Check sheet for the modelled part. Datum: model origin and axes. Units: mm. A direction names the side the tool comes from. Coordinates: 2 decimals unless noted, no trailing zeros. Loops run counter-clockwise (first coordinate to the right, second up) from the corner with the lowest first, then second, coordinate; pieces in that order, holes last. Notation, with made-up numbers: M 75,17 L 113,17 A22 ccw 113,33 Z; hole C 36.5,-29 d9. An arc over 180 degrees is marked long. Return JSON: item names as keys, results as strings.
from build123d import *

# Parameters (mm, degrees)
SKETCH1_W           = 10.6496793
SKETCH1_H           = 5.5
SKETCH1_W_2         = 3
SKETCH1_H_2         = 45
BOSS_EXTRUDE1_DEPTH = 80
SKETCH2_R           = 2
SKETCH2_R_2         = 1.25
CUT_EXTRUDE1_DEPTH  = 87.830296046
SKETCH3_R           = 5
SKETCH3_R_2         = 1.0922
CUT_EXTRUDE2_DEPTH  = 10
SKETCH4_W           = 28
SKETCH4_H           = 3
SKETCH4_W_2         = 8.5
BOSS_EXTRUDE2_DEPTH = 10.6496793


with BuildPart() as part:
    # Sketch1 → Boss-Extrude1 (new body)
    with BuildSketch(Plane(origin=(0, 0, 0), x_dir=(1, 0, 0), z_dir=(0, 1, 0))):
        with Locations((8.035561223, -6.751971663)):
            Rectangle(SKETCH1_W, SKETCH1_H)
        with Locations((1.210721573, 4.498028337)):
            Rectangle(SKETCH1_W_2, SKETCH1_H_2)
        with Locations((8.035561223, -15.251971663)):
            Rectangle(SKETCH1_W, SKETCH1_H)
    extrude(amount=BOSS_EXTRUDE1_DEPTH)

    # Sketch2 → Cut-Extrude1 (cut, through all)
    with BuildSketch(Plane(origin=(0, 0, 4.001971663), x_dir=(-1, 0, 0), z_dir=(0, 0, -1))):
        with Locations((-7.660400873, 40)):
            Circle(SKETCH2_R)
        with Locations((-7.660400873, 65.273758001)):
            Circle(SKETCH2_R_2)
        with Locations((-7.660400873, 14.726241999)):
            Circle(SKETCH2_R_2)
    extrude(amount=-CUT_EXTRUDE1_DEPTH, mode=Mode.SUBTRACT)

    # Sketch3 → Cut-Extrude2 (cut)
    with BuildSketch(Plane(origin=(2.710721573, 0, 0), x_dir=(0, 0, -1), z_dir=(1, 0, 0))):
        with Locations((7.298028337, 40)):
            Circle(SKETCH3_R)
        with Locations((7.298028337, 74.25)):
            Circle(SKETCH3_R_2)
        with Locations((7.298028337, 5.75)):
            Circle(SKETCH3_R_2)
    extrude(amount=-CUT_EXTRUDE2_DEPTH, mode=Mode.SUBTRACT)

    # Sketch4 → Boss-Extrude2 (add)
    with BuildSketch(Plane(origin=(2.710721573, 0, 0), x_dir=(0, 0, -1), z_dir=(1, 0, 0))):
        Polygon((26.998028337, 0), (26.998028337, 80), (23.998028337, 80), (23.998028337, 77), (23.998028337, 3), (23.998028337, 0), align=None)
        with Locations((9.998028337, 78.5)):
            Rectangle(SKETCH4_W, SKETCH4_H)
        with Locations((9.998028337, 1.5)):
            Rectangle(SKETCH4_W, SKETCH4_H)
        with Locations((-8.251971663, 78.5)):
            Rectangle(SKETCH4_W_2, SKETCH4_H)
        with Locations((-8.251971663, 1.5)):
            Rectangle(SKETCH4_W_2, SKETCH4_H)
    extrude(amount=BOSS_EXTRUDE2_DEPTH)


solid = part.part
1) Set-up check for faces 1 (the face through (8, 77, -10)), 2 (the face through (6.468, 15.102, 6.713)), 3 (the face through (6, 80, -5)): record each of +Z, -Z, +X, -X, +Y, -Y from which the full face is reachable in a straight line by a thin tool's end or side.
Answers:
{"face 1": "+X", "face 2": "+Z", "face 3": "+Z, -Z, +X, -X, +Y"}
2) Scan lines: line 1 along Z through (x, y) = (11.75, 14.5); line 2 along Y through (x, z) = (11.5, -20); line 3 along Y through (x, z) = (2, -3). Record each from-to range of solid material in increasing order. Write a range as [from, to].
Answers:
{"line 1": "[-27, -24], [4, 9.5], [12.5, 18]", "line 2": "[0, 3], [77, 80]", "line 3": "[0, 37.45], [42.55, 80]"}
3) Section check D-D on x = 0.5. Record the cut outline in (y, z).
Answers:
{"outline": "M 0,-27 L 80,-27 L 80,18 L 0,18 Z; hole C 5.75,-7.3 d2.18; hole C 40,-7.3 d10; hole C 74.25,-7.3 d2.18"}
4) Go/stop test with flat-tipped pins: pin 1 Ø0.9 at (y, z) = (56, 11) entering from +X; pin 2 Ø9 at (y, z) = (40, -7.3) entering from -X. Record where each tip stops, or that it passes through.
Answers:
{"pin 1": "x = 2.71", "pin 2": "through"}
5) Section check C-C on y = 5.75. Record the cut outline in (x, z), then the cut area to 3 significant figures.
Answers:
{"outline": "M -0.29,-27 L 13.36,-27 L 13.36,-24 L 2.71,-24 L 2.71,-8.39 L -0.29,-8.39 Z; M -0.29,-6.21 L 2.71,-6.21 L 2.71,4 L 13.36,4 L 13.36,9.5 L 2.71,9.5 L 2.71,12.5 L 13.36,12.5 L 13.36,18 L -0.29,18 Z", "area": "278 mm²"}
6) Draft check along Z on faces 4 (the face through (1.232, 5.798, -6.207)), 5 (the face through (8, 77, 11)), 6 (the face through (8.094, 38.048, 15.213)), 7 (the face through (6, 39, -26.998)). Enter one of: +Z half, -Z half, draft (parallel to the pull), parting line (faces both ways), or undercut.
Answers:
{"face 4": "undercut", "face 5": "undercut", "face 6": "draft", "face 7": "-Z half"}
7) Section check A-A on y = 40. Record the cut outline in (x, z), then the cut area to 3 significant figures.
Answers:
{"outline": "M -0.29,-27 L 13.36,-27 L 13.36,-24 L 2.71,-24 L 2.71,-12.3 L -0.29,-12.3 Z; M -0.29,-2.3 L 2.71,-2.3 L 2.71,4 L 5.66,4 L 5.66,9.5 L 2.71,9.5 L 2.71,12.5 L 5.66,12.5 L 5.66,18 L -0.29,18 Z; M 9.66,4 L 13.36,4 L 13.36,9.5 L 9.66,9.5 Z; M 9.66,12.5 L 13.36,12.5 L 13.36,18 L 9.66,18 Z", "area": "210 mm²"}
8) Section check B-B on x = 11.5. Record the cut outline in (y, z), then the cut area to 3 significant figures.
Answers:
{"outline": "M 0,-27 L 80,-27 L 80,18 L 0,18 Z; hole M 3,-24 L 77,-24 L 77,4 L 3,4 Z; hole M 3,9.5 L 77,9.5 L 77,12.5 L 3,12.5 Z", "area": "1,310 mm²"}
